from build123d import *

# Parameters (mm, degrees)
SKETCH1_W           = 3
SKETCH1_H           = 4.5
BOSS_EXTRUDE1_DEPTH = 3


with BuildPart() as part:
    # Sketch1 → Boss-Extrude1 (new body)
    with BuildSketch(Plane.XY):
        with BuildLine():
            Line((187.5, 3), (187.5, 6))
            Line((187.5, 6), (184.5, 6))
            Line((184.5, 6), (184.5, 3))
            Line((184.5, 3), (175.5, 3))
            Line((175.5, 3), (175.5, 6))
            Line((175.5, 6), (172.5, 6))
            Line((172.5, 6), (172.5, 3))
            Line((172.5, 3), (163.5, 3))
            Line((163.5, 3), (163.5, 6))
            Line((163.5, 6), (160.5, 6))
            Line((160.5, 6), (160.5, 3))
            Line((160.5, 3), (151.5, 3))
            Line((151.5, 3), (151.5, 6))
            Line((151.5, 6), (148.5, 6))
            Line((148.5, 6), (148.5, 3))
            Line((148.5, 3), (139.5, 3))
            Line((139.5, 3), (139.5, 6))
            Line((139.5, 6), (136.5, 6))
            Line((136.5, 6), (136.5, 3))
            Line((136.5, 3), (127.5, 3))
            Line((127.5, 3), (127.5, 6))
            Line((127.5, 6), (124.5, 6))
            Line((124.5, 6), (124.5, 3))
            Line((124.5, 3), (115.5, 3))
            Line((115.5, 3), (115.5, 6))
            Line((115.5, 6), (112.5, 6))
            Line((112.5, 6), (112.5, 3))
            Line((112.5, 3), (103.5, 3))
            Line((103.5, 3), (103.5, 6))
            Line((103.5, 6), (100.5, 6))
            Line((100.5, 6), (100.5, 3))
            Line((100.5, 3), (91.5, 3))
            Line((91.5, 3), (91.5, 6))
            Line((91.5, 6), (88.5, 6))
            Line((88.5, 6), (88.5, 3))
            Line((88.5, 3), (79.5, 3))
            Line((79.5, 3), (79.5, 6))
            Line((79.5, 6), (76.5, 6))
            Line((76.5, 6), (76.5, 3))
            Line((76.5, 3), (67.5, 3))
            Line((67.5, 3), (67.5, 6))
            Line((67.5, 6), (64.5, 6))
            Line((64.5, 6), (64.5, 3))
            Line((64.5, 3), (55.5, 3))
            Line((55.5, 3), (55.5, 6))
            Line((55.5, 6), (52.5, 6))
            Line((52.5, 6), (52.5, 3))
            Line((52.5, 3), (43.5, 3))
            Line((43.5, 3), (43.5, 6))
            Line((43.5, 6), (40.5, 6))
            Line((40.5, 6), (40.5, 3))
            Line((40.5, 3), (31.5, 3))
            Line((31.5, 3), (31.5, 6))
            Line((31.5, 6), (28.5, 6))
            Line((28.5, 6), (28.5, 3))
            Line((28.5, 3), (19.5, 3))
            Line((19.5, 3), (19.5, 6))
            Line((19.5, 6), (16.5, 6))
            Line((16.5, 6), (16.5, 3))
            Line((16.5, 3), (13.5, 3))
            Line((13.5, 3), (13.5, 10.5))
            Line((13.5, 10.5), (10.5, 10.5))
            Line((10.5, 10.5), (10.5, 3))
            Line((10.5, 3), (7.5, 6))
            ThreePointArc((7.5, 6), (6.312305899, 11.031152949), (3, 15))
            Line((3, 15), (22.5, 15))
            Line((22.5, 15), (22.5, 18))
            Line((22.5, 18), (25.5, 18))
            Line((25.5, 18), (25.5, 15))
            Line((25.5, 15), (70.5, 15))
            Line((70.5, 15), (70.5, 18))
            Line((70.5, 18), (73.5, 18))
            Line((73.5, 18), (73.5, 15))
            Line((73.5, 15), (142.5, 15))
            Line((142.5, 15), (142.5, 18))
            Line((142.5, 18), (145.5, 18))
            Line((145.5, 18), (145.5, 15))
            Line((145.5, 15), (190.5, 15))
            Line((190.5, 15), (190.5, 18))
            Line((190.5, 18), (193.5, 18))
            Line((193.5, 18), (193.5, 15))
            Line((193.5, 15), (202.5, 15))
            Line((202.5, 15), (202.5, 10.5))
            Line((202.5, 10.5), (205.5, 10.5))
            Line((205.5, 10.5), (205.5, 15))
            Line((205.5, 15), (213, 15))
            ThreePointArc((213, 15), (209.687694101, 11.031152949), (208.5, 6))
            Line((208.5, 6), (205.5, 3))
            Line((205.5, 3), (199.5, 3))
            Line((199.5, 3), (199.5, 6))
            Line((199.5, 6), (196.5, 6))
            Line((196.5, 6), (196.5, 3))
            Line((196.5, 3), (187.5, 3))
        make_face()
        with Locations((24, 8.25)):
            Rectangle(SKETCH1_W, SKETCH1_H, mode=Mode.SUBTRACT)
        with Locations((36, 8.25)):
            Rectangle(SKETCH1_W, SKETCH1_H, mode=Mode.SUBTRACT)
        with Locations((48, 8.25)):
            Rectangle(SKETCH1_W, SKETCH1_H, mode=Mode.SUBTRACT)
        with Locations((60, 8.25)):
            Rectangle(SKETCH1_W, SKETCH1_H, mode=Mode.SUBTRACT)
        with Locations((72, 8.25)):
            Rectangle(SKETCH1_W, SKETCH1_H, mode=Mode.SUBTRACT)
        with Locations((84, 8.25)):
            Rectangle(SKETCH1_W, SKETCH1_H, mode=Mode.SUBTRACT)
        with Locations((96, 8.25)):
            Rectangle(SKETCH1_W, SKETCH1_H, mode=Mode.SUBTRACT)
        with Locations((108, 8.25)):
            Rectangle(SKETCH1_W, SKETCH1_H, mode=Mode.SUBTRACT)
        with Locations((120, 8.25)):
            Rectangle(SKETCH1_W, SKETCH1_H, mode=Mode.SUBTRACT)
        with Locations((132, 8.25)):
            Rectangle(SKETCH1_W, SKETCH1_H, mode=Mode.SUBTRACT)
        with Locations((144, 8.25)):
            Rectangle(SKETCH1_W, SKETCH1_H, mode=Mode.SUBTRACT)
        with Locations((156, 8.25)):
            Rectangle(SKETCH1_W, SKETCH1_H, mode=Mode.SUBTRACT)
        with Locations((168, 8.25)):
            Rectangle(SKETCH1_W, SKETCH1_H, mode=Mode.SUBTRACT)
        with Locations((180, 8.25)):
            Rectangle(SKETCH1_W, SKETCH1_H, mode=Mode.SUBTRACT)
        with Locations((192, 8.25)):
            Rectangle(SKETCH1_W, SKETCH1_H, mode=Mode.SUBTRACT)
    extrude(amount=BOSS_EXTRUDE1_DEPTH)


solid = part.part
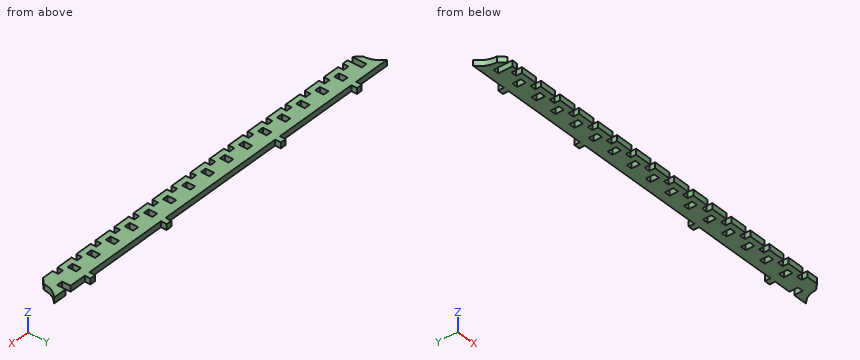
Work out the finished part from the listing and answer in its coordinate system (mm). Round coordinates to 2 decimals unless told otherwise and drop trailing zeros. Write each loop counter-clockwise with the first axis right and the second up, starting at its lowest first coordinate (ties: lowest second). Pieces come first, ordered by that corner, then holes.
1) A cutting plane is placed at B-B (z = 1.2). Give the number of separate pieces and of enclosed holes in the cut face, plus the area to 3 significant figures.
2) Given pin 1 Ø0.9 at (x, z) = (108.5, 1.5) entering from +Y; pin 2 Ø0.9 at (y, z) = (8, 2) entering from -X, each flat-ended and moving along its own axis, determine where each tip first touches the part or whether it passes through.
3) A cutting plane is placed at A-A (y = 12.5). Give the vertices of the cut face in (x, z).
4) Straight lines are drawn through the part: line 1 (X direction, y = 16.25, z = 2); line 2 (Y direction, x = 107, z = 0.8); line 3 (X direction, y = 12.5, z = 1.6). For each, find the intervals that lie inside material, in ascending order.
Completed:
1. separate pieces: 1
1. enclosed holes: 15
1. area: 2,080 mm2
2. pin 1: stops at y = 15
2. pin 2: stops at x = 7.23
3. outline: (5.43, 0) - (202.5, 0) - (202.5, 3) - (5.43, 3) - close; (205.5, 0) - (210.57, 0) - (210.57, 3) - (205.5, 3) - close
4. line 1: x = 22.5 to 25.5, 70.5 to 73.5, 142.5 to 145.5, 190.5 to 193.5
4. line 2: y = 3 to 6, 10.5 to 15
4. line 3: x = 5.43 to 202.5, 205.5 to 210.57
